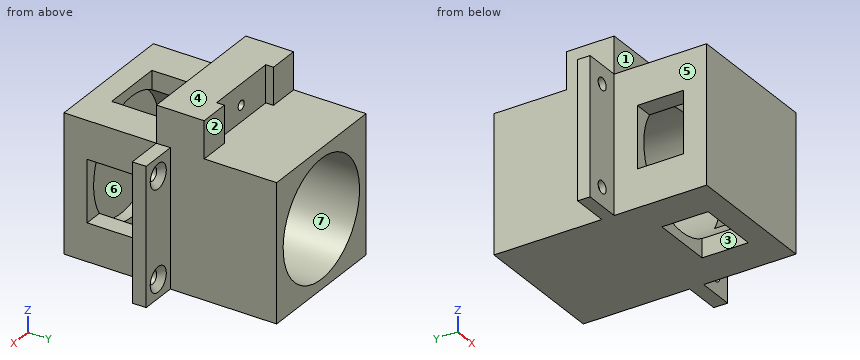
from build123d import *

# Parameters (mm, degrees)
SKETCH1_W                     = 44.45
SKETCH1_H                     = 44.45
BOSS_EXTRUDE1_DEPTH           = 90
SKETCH2_R                     = 19
CUT_EXTRUDE1_DEPTH            = 45
SKETCH3_R                     = 19
CUT_EXTRUDE2_DEPTH            = 41
SKETCH4_W                     = 44.45
SKETCH4_H                     = 44.45
CUT_EXTRUDE3_DEPTH            = 21
SKETCH6_W                     = 20
SKETCH6_H                     = 15
CUT_EXTRUDE4_DEPTH            = 86.033835178
SKETCH8_W                     = 20
SKETCH8_H                     = 15
CUT_EXTRUDE5_DEPTH            = 86.033835178
BOSS_EXTRUDE2_DEPTH           = 12
SKETCH20_R                    = 1.51
CUT_EXTRUDE6_DEPTH            = 13
SKETCH21_W                    = 44.45
SKETCH21_H                    = 4
BOSS_EXTRUDE4_DEPTH           = 12
SKETCH22_R                    = 4
CUT_EXTRUDE11_DEPTH           = 2
CUT_EXTRUDE11_DRAFT           = -45
CUT_EXTRUDE11_PROFILE_2_DEPTH = 2
CUT_EXTRUDE11_PROFILE_2_DRAFT = -45
CUT_EXTRUDE11_PROFILE_3_DEPTH = 2
CUT_EXTRUDE11_PROFILE_3_DRAFT = -45
CUT_EXTRUDE11_PROFILE_4_DEPTH = 2
CUT_EXTRUDE11_PROFILE_4_DRAFT = -45
SKETCH23_R                    = 2
CUT_EXTRUDE12_DEPTH           = 12
SKETCH24_W                    = 44.45
SKETCH24_H                    = 4.5
BOSS_EXTRUDE5_DEPTH           = 12
SKETCH25_R                    = 4
CUT_EXTRUDE13_DEPTH           = 2
CUT_EXTRUDE13_DRAFT           = -45
CUT_EXTRUDE13_PROFILE_2_DEPTH = 2
CUT_EXTRUDE13_PROFILE_2_DRAFT = -45
SKETCH26_R                    = 2.125
CUT_EXTRUDE14_DEPTH           = 12


with BuildPart() as part:
    # Sketch1 → Boss-Extrude1 (new body)
    with BuildSketch(Plane(origin=(0, 0, 0), x_dir=(1, 0, 0), z_dir=(0, 1, 0))):
        Rectangle(SKETCH1_W, SKETCH1_H)
    extrude(amount=BOSS_EXTRUDE1_DEPTH)

    # Sketch2 → Cut-Extrude1 (cut)
    with BuildSketch(Plane(origin=(0, 90, 0), x_dir=(1, 0, 0), z_dir=(0, 1, 0))):
        with Locations(Location((0, 0, 0), (0, 0, 270))):
            Circle(SKETCH2_R)
    extrude(amount=-CUT_EXTRUDE1_DEPTH, mode=Mode.SUBTRACT)

    # Sketch3 → Cut-Extrude2 (cut)
    with BuildSketch(Plane(origin=(0, 45, 0), x_dir=(1, 0, 0), z_dir=(0, 1, 0))):
        with Locations(Location((0, 0, 0), (0, 0, 270))):
            Circle(SKETCH3_R)
    extrude(amount=-CUT_EXTRUDE2_DEPTH, mode=Mode.SUBTRACT)

    # Sketch4 → Cut-Extrude3 (cut)
    with BuildSketch(Plane(origin=(0, 90, 0), x_dir=(1, 0, 0), z_dir=(0, 1, 0))):
        Rectangle(SKETCH4_W, SKETCH4_H)
    extrude(amount=-CUT_EXTRUDE3_DEPTH, mode=Mode.SUBTRACT)

    # Sketch6 → Cut-Extrude4 (cut, through all)
    with BuildSketch(Plane.XY.offset(22.225)):
        with Locations((0, 15)):
            Rectangle(SKETCH6_W, SKETCH6_H)
    extrude(amount=-CUT_EXTRUDE4_DEPTH, mode=Mode.SUBTRACT)

    # Sketch8 → Cut-Extrude5 (cut, through all)
    with BuildSketch(Plane.ZY.offset(22.225)):
        with Locations((0, 15)):
            Rectangle(SKETCH8_W, SKETCH8_H)
    extrude(amount=-CUT_EXTRUDE5_DEPTH, mode=Mode.SUBTRACT)

    # Sketch18 → Boss-Extrude2 (add)
    with BuildSketch(Plane.XY.offset(22.225)):
        Polygon((12.2, 45.5), (22.225, 45.5), (22.225, 30), (-22.225, 30), (-22.225, 45.5), (-12.2, 45.5), (-12.2, 43), (12.2, 43), align=None)
    extrude(amount=BOSS_EXTRUDE2_DEPTH)

    # Sketch20 → Cut-Extrude6 (cut)
    with BuildSketch(Plane(origin=(0, 43, 0), x_dir=(1, 0, 0), z_dir=(0, 1, 0))):
        with Locations(Location((0, -27.475, 0), (0, 0, 270))):
            Circle(SKETCH20_R)
    extrude(amount=-CUT_EXTRUDE6_DEPTH, mode=Mode.SUBTRACT)

    # Sketch21 → Boss-Extrude4 (add)
    with BuildSketch(Plane.ZY.offset(22.225)):
        with Locations((0, 32)):
            Rectangle(SKETCH21_W, SKETCH21_H)
    extrude(amount=BOSS_EXTRUDE4_DEPTH)


with BuildPart() as cut_extrude11_tool:
    # Sketch22 → Cut-Extrude11 (with draft: the straight prism first)
    with BuildSketch(Plane(origin=(0, 34, 0), x_dir=(1, 0, 0), z_dir=(0, 1, 0))):
        with Locations((-28.225, -16.225)):
            Circle(SKETCH22_R)
    extrude(amount=-CUT_EXTRUDE11_DEPTH)
    # Cut-Extrude11: the draft: its side faces are tilted about the plane it starts from
    cut_extrude11_sides = [cut_extrude11_tool.faces().sort_by_distance(p)[0] for p in [
        (-32.225, 33, 16.225),
    ]]
    draft(cut_extrude11_sides, Plane(origin=(0, 34, 0), x_dir=(1, 0, 0), z_dir=(0, 1, 0)), CUT_EXTRUDE11_DRAFT)


with BuildPart() as part_1:
    add(part.part)

    # Cut-Extrude11: cut by cut_extrude11_tool
    add(cut_extrude11_tool.part, mode=Mode.SUBTRACT)


with BuildPart() as cut_extrude11_profile_2_tool:
    # Sketch22 → Cut-Extrude11 profile 2 (with draft: the straight prism first)
    with BuildSketch(Plane(origin=(0, 34, 0), x_dir=(1, 0, 0), z_dir=(0, 1, 0))):
        with Locations((-28.225, 16.225)):
            Circle(SKETCH22_R)
    extrude(amount=-CUT_EXTRUDE11_PROFILE_2_DEPTH)
    # Cut-Extrude11 profile 2: the draft: its side faces are tilted about the plane it starts from
    cut_extrude11_profile_2_sides = [cut_extrude11_profile_2_tool.faces().sort_by_distance(p)[0] for p in [
        (-32.225, 33, -16.225),
    ]]
    draft(cut_extrude11_profile_2_sides, Plane(origin=(0, 34, 0), x_dir=(1, 0, 0), z_dir=(0, 1, 0)), CUT_EXTRUDE11_PROFILE_2_DRAFT)


with BuildPart() as part_2:
    add(part_1.part)

    # Cut-Extrude11 profile 2: cut by cut_extrude11_profile_2_tool
    add(cut_extrude11_profile_2_tool.part, mode=Mode.SUBTRACT)


with BuildPart() as cut_extrude11_profile_3_tool:
    # Sketch22 → Cut-Extrude11 profile 3 (with draft: the straight prism first)
    with BuildSketch(Plane(origin=(0, 34, 0), x_dir=(1, 0, 0), z_dir=(0, 1, 0))):
        with Locations((28.225, -16.225)):
            Circle(SKETCH22_R)
    extrude(amount=-CUT_EXTRUDE11_PROFILE_3_DEPTH)
    # Cut-Extrude11 profile 3: the draft: its side faces are tilted about the plane it starts from
    cut_extrude11_profile_3_sides = [cut_extrude11_profile_3_tool.faces().sort_by_distance(p)[0] for p in [
        (24.225, 33, 16.225),
    ]]
    draft(cut_extrude11_profile_3_sides, Plane(origin=(0, 34, 0), x_dir=(1, 0, 0), z_dir=(0, 1, 0)), CUT_EXTRUDE11_PROFILE_3_DRAFT)


with BuildPart() as part_3:
    add(part_2.part)

    # Cut-Extrude11 profile 3: cut by cut_extrude11_profile_3_tool
    add(cut_extrude11_profile_3_tool.part, mode=Mode.SUBTRACT)


with BuildPart() as cut_extrude11_profile_4_tool:
    # Sketch22 → Cut-Extrude11 profile 4 (with draft: the straight prism first)
    with BuildSketch(Plane(origin=(0, 34, 0), x_dir=(1, 0, 0), z_dir=(0, 1, 0))):
        with Locations((28.225, 16.225)):
            Circle(SKETCH22_R)
    extrude(amount=-CUT_EXTRUDE11_PROFILE_4_DEPTH)
    # Cut-Extrude11 profile 4: the draft: its side faces are tilted about the plane it starts from
    cut_extrude11_profile_4_sides = [cut_extrude11_profile_4_tool.faces().sort_by_distance(p)[0] for p in [
        (24.225, 33, -16.225),
    ]]
    draft(cut_extrude11_profile_4_sides, Plane(origin=(0, 34, 0), x_dir=(1, 0, 0), z_dir=(0, 1, 0)), CUT_EXTRUDE11_PROFILE_4_DRAFT)


with BuildPart() as part_4:
    add(part_3.part)

    # Cut-Extrude11 profile 4: cut by cut_extrude11_profile_4_tool
    add(cut_extrude11_profile_4_tool.part, mode=Mode.SUBTRACT)

    # Sketch23 → Cut-Extrude12 (cut)
    with BuildSketch(Plane(origin=(0, 34, 0), x_dir=(1, 0, 0), z_dir=(0, 1, 0))):
        with Locations(Location((-28.225, -16.225, 0), (0, 0, 270))):
            Circle(SKETCH23_R)
        with Locations(Location((-28.225, 16.225, 0), (0, 0, 90))):
            Circle(SKETCH23_R)
    extrude(amount=-CUT_EXTRUDE12_DEPTH, mode=Mode.SUBTRACT)

    # Sketch24 → Boss-Extrude5 (add)
    with BuildSketch(Plane(origin=(22.225, 0, 0), x_dir=(0, 0, -1), z_dir=(1, 0, 0))):
        with Locations((0, 32.25)):
            Rectangle(SKETCH24_W, SKETCH24_H)
    extrude(amount=BOSS_EXTRUDE5_DEPTH)


with BuildPart() as cut_extrude13_tool:
    # Sketch25 → Cut-Extrude13 (with draft: the straight prism first)
    with BuildSketch(Plane(origin=(0, 34.5, 0), x_dir=(1, 0, 0), z_dir=(0, 1, 0))):
        with Locations((28.225, 16.225)):
            Circle(SKETCH25_R)
    extrude(amount=-CUT_EXTRUDE13_DEPTH)
    # Cut-Extrude13: the draft: its side faces are tilted about the plane it starts from
    cut_extrude13_sides = [cut_extrude13_tool.faces().sort_by_distance(p)[0] for p in [
        (24.225, 33.5, -16.225),
    ]]
    draft(cut_extrude13_sides, Plane(origin=(0, 34.5, 0), x_dir=(1, 0, 0), z_dir=(0, 1, 0)), CUT_EXTRUDE13_DRAFT)


with BuildPart() as part_5:
    add(part_4.part)

    # Cut-Extrude13: cut by cut_extrude13_tool
    add(cut_extrude13_tool.part, mode=Mode.SUBTRACT)


with BuildPart() as cut_extrude13_profile_2_tool:
    # Sketch25 → Cut-Extrude13 profile 2 (with draft: the straight prism first)
    with BuildSketch(Plane(origin=(0, 34.5, 0), x_dir=(1, 0, 0), z_dir=(0, 1, 0))):
        with Locations((28.225, -16.225)):
            Circle(SKETCH25_R)
    extrude(amount=-CUT_EXTRUDE13_PROFILE_2_DEPTH)
    # Cut-Extrude13 profile 2: the draft: its side faces are tilted about the plane it starts from
    cut_extrude13_profile_2_sides = [cut_extrude13_profile_2_tool.faces().sort_by_distance(p)[0] for p in [
        (24.225, 33.5, 16.225),
    ]]
    draft(cut_extrude13_profile_2_sides, Plane(origin=(0, 34.5, 0), x_dir=(1, 0, 0), z_dir=(0, 1, 0)), CUT_EXTRUDE13_PROFILE_2_DRAFT)


with BuildPart() as part_6:
    add(part_5.part)

    # Cut-Extrude13 profile 2: cut by cut_extrude13_profile_2_tool
    add(cut_extrude13_profile_2_tool.part, mode=Mode.SUBTRACT)

    # Sketch26 → Cut-Extrude14 (cut)
    with BuildSketch(Plane(origin=(0, 34.5, 0), x_dir=(1, 0, 0), z_dir=(0, 1, 0))):
        with Locations(Location((28.225, 16.225, 0), (0, 0, 270))):
            Circle(SKETCH26_R)
        with Locations(Location((28.225, -16.225, 0), (0, 0, 270))):
            Circle(SKETCH26_R)
    extrude(amount=-CUT_EXTRUDE14_DEPTH, mode=Mode.SUBTRACT)


solid = part_6.part
Read the model definition and answer for the solid it produces. Units are mm, in the model's axes. Face numbers are marked on the shaded views. A direction names the side the tool comes from. Give positions to 0.01 mm unless a question says otherwise; leave off trailing zeros. Write each loop counter-clockwise with the first axis right and the second up, starting at its lowest first coordinate (ties: lowest second). Pieces come first, ordered by that corner, then holes. Notation, with made-up numbers: (70.25, 67.5) - (92.25, 67.5) arc R21 cw to (92.25, 93.5) - close; hole circle Ø8 at (84.5, -1). An arc over 180 degrees is marked (long way). Answer in a Markdown table with one row per item. Add a question column.
Item 1: Section C-C, the plane y = 10 is taken. Write down the section's boundary in (x, z) (1 decimal).
Item 2: Find the intervals of material crossed by L1, parallel to Y at x = -18.5, z = 7.5; L2, parallel to Y at x = -4.5, z = 8.5; L3, parallel to X at y = 44.5, z = 0 (3 decimals), in increasing order.
Item 3: A tool of negligible diameter and unlimited length cuts with its end or side. For the marked faces 1, 2 and 3, from which of +Z, -Z, +X, -X, +Y, -Y can it reach the whole face along a straight path? Write none if from no direction.
Item 4: Flat-ended cylindrical pins translate along their axes: P1, Ø1, axis at x = -11, z = -1, coming from the +Y side; P2, Ø9, axis at y = 10, z = 3, coming from the +X side (3 decimals); P3, Ø9, axis at y = 8.5, z = 8.5, coming from the -X side (3 decimals); P4, Ø3.5, axis at x = 28.225, z = 16.225, coming from the -Y side. Find the tip coordinate at first contact, or state that the pin passes through.
Item 5: Determine the mould class of the marked faces 4, 5, 6 and 7 for opening direction Z: pulls with the +Z half, pulls with the -Z half, needs draft (parallel to the pull), parting line crosses it, or undercut.
Item 6: Section A-A, the plane z = 0 is taken. Write down the section's boundary in (x, y) (3 decimals), and give its area (3 significant figures).
Item 7: Section B-B, the plane x = 0 is taken. Write down the section's boundary in (y, z) (3 decimals), and give its area (3 significant figures).
Item 8: Section D-D, the plane x = -7 is taken. Write down the section's boundary in (y, z) (3 decimals).
Recorded:
| question | item | result |
|---|---|---|
| 1 | outline | (-22.2, -22.2) - (-10, -22.2) - (-10, -16.2) arc R19 cw to (-16.2, -10) - (-22.2, -10) - close; (-22.2, 10) - (-16.2, 10) arc R19 cw to (-10, 16.2) - (-10, 22.2) - (-22.2, 22.2) - close; (10, -22.2) - (22.2, -22.2) - (22.2, -10) - (16.2, -10) arc R19 cw to (10, -16.2) - close; (10, 16.2) arc R19 cw to (16.2, 10) - (22.2, 10) - (22.2, 22.2) - (10, 22.2) - close |
| 2 | L1 | y = 0 to 7.5, 22.5 to 69 |
| 2 | L2 | y = 0 to 4 |
| 2 | L3 | x = -22.225 to -19, 19 to 22.225 |
| 3 | face 1 | +Z, +X, -X, -Y |
| 3 | face 2 | +Z, +X, -X, +Y |
| 3 | face 3 | +Z, -Z |
| 4 | P1 | stops at y = 4 |
| 4 | P2 | stops at x = 22.225 |
| 4 | P3 | stops at x = -22.225 |
| 4 | P4 | passes through |
| 5 | face 4 | pulls with the +Z half |
| 5 | face 5 | needs draft |
| 5 | face 6 | undercut |
| 5 | face 7 | undercut |
| 6 | outline | (-34.225, 30) - (-22.225, 30) - (-22.225, 22.5) - (-19, 22.5) - (-19, 69) - (-22.225, 69) - (-22.225, 34) - (-34.225, 34) - close; (-22.225, 0) - (22.225, 0) - (22.225, 7.5) - (19, 7.5) - (19, 4) - (-19, 4) - (-19, 7.5) - (-22.225, 7.5) - close; (19, 22.5) - (22.225, 22.5) - (22.225, 30) - (34.225, 30) - (34.225, 34.5) - (22.225, 34.5) - (22.225, 69) - (19, 69) - close |
| 6 | area | 602 mm2 |
| 7 | outline | (0, -22.225) - (7.5, -22.225) - (7.5, -19) - (4, -19) - (4, 19) - (7.5, 19) - (7.5, 22.225) - (0, 22.225) - close; (22.5, -22.225) - (69, -22.225) - (69, -19) - (22.5, -19) - close; (22.5, 19) - (69, 19) - (69, 22.225) - (43, 22.225) - (43, 25.965) - (30, 25.965) - (30, 22.225) - (22.5, 22.225) - close; (30, 28.985) - (43, 28.985) - (43, 34.225) - (30, 34.225) - close |
| 7 | area | 617 mm2 |
| 8 | outline | (0, -22.225) - (7.5, -22.225) - (7.5, -17.664) - (4, -17.664) - (4, 17.664) - (7.5, 17.664) - (7.5, 22.225) - (0, 22.225) - close; (22.5, -22.225) - (69, -22.225) - (69, -17.664) - (22.5, -17.664) - close; (22.5, 17.664) - (69, 17.664) - (69, 22.225) - (43, 22.225) - (43, 34.225) - (30, 34.225) - (30, 22.225) - (22.5, 22.225) - close |
